```python
from build123d import *
from OCP.BRepFilletAPI import BRepFilletAPI_MakeChamfer

# Parameters (mm, degrees)
SKETCH2_W           = 152.4
SKETCH2_H           = 152.4
BOSS_EXTRUDE1_DEPTH = 25.4
BOSS_EXTRUDE2_DEPTH = 101.6
BOSS_EXTRUDE5_START = 50.8
BOSS_EXTRUDE5_DEPTH = 50.8
BOSS_EXTRUDE6_DEPTH = 25.4
SKETCH6_W           = 127
SKETCH6_H           = 98.02354915
CUT_EXTRUDE1_DEPTH  = 139.7
SKETCH7_R           = 8.255
CUT_EXTRUDE2_DEPTH  = 12.7
CHAMFER1_SIZE       = 7.62
CHAMFER1_SIZE2      = 2.773453185
FILLET1_R           = 12.7


with BuildPart() as part:
    # Sketch2 → Boss-Extrude1 (new body)
    with BuildSketch(Plane(origin=(0, 0, 0), x_dir=(1, 0, 0), z_dir=(0, 1, 0))):
        with BuildLine():
            Line((0, 76.2), (76.2, 76.2))
            Line((76.2, 76.2), (76.2, 123.42354915))
            ThreePointArc((76.2, 123.42354915), (44.823274072, 88.963087986), (0, 76.2))
        make_face()
        with BuildLine():
            Line((-76.2, 123.42354915), (-76.2, 76.2))
            Line((-76.2, 76.2), (0, 76.2))
            ThreePointArc((0, 76.2), (-44.823274072, 88.963087986), (-76.2, 123.42354915))
        make_face()
        Rectangle(SKETCH2_W, SKETCH2_H)
    extrude(amount=BOSS_EXTRUDE1_DEPTH)

    # Sketch3 → Boss-Extrude2 (add)
    with BuildSketch(Plane(origin=(0, 25.4, 0), x_dir=(1, 0, 0), z_dir=(0, 1, 0))):
        with BuildLine():
            ThreePointArc((76.2, 123.42354915), (0, 76.2), (-76.2, 123.42354915))
            Line((-76.2, 123.42354915), (-76.2, 98.02354915))
            ThreePointArc((-76.2, 98.02354915), (0, 60.787742764), (76.2, 98.02354915))
            Line((76.2, 98.02354915), (76.2, 123.42354915))
        make_face()
        with BuildLine():
            ThreePointArc((76.2, 78.97354915), (0, 46.95399651), (-76.2, 78.97354915))
            Line((-76.2, 78.97354915), (-76.2, -76.2))
            Line((-76.2, -76.2), (76.2, -76.2))
            Line((76.2, -76.2), (76.2, 78.97354915))
        make_face()
    extrude(amount=BOSS_EXTRUDE2_DEPTH)

    # Sketch5 → Boss-Extrude5 (add)
    with BuildSketch(Plane(origin=(0, 0, 0), x_dir=(1, 0, 0), z_dir=(0, 1, 0)).offset(BOSS_EXTRUDE5_START)):
        with BuildLine():
            Line((-76.2, 123.42354915), (-76.2, -76.2))
            Line((-76.2, -76.2), (76.2, -76.2))
            Line((76.2, -76.2), (76.2, 123.42354915))
            ThreePointArc((76.2, 123.42354915), (0, 76.2), (-76.2, 123.42354915))
        make_face()
    extrude(amount=BOSS_EXTRUDE5_DEPTH)

    # Sketch4 → Boss-Extrude6 (add)
    with BuildSketch(Plane(origin=(0, 127, 0), x_dir=(1, 0, 0), z_dir=(0, 1, 0))):
        with BuildLine():
            Line((-76.2, 123.42354915), (-76.2, -76.2))
            Line((-76.2, -76.2), (76.2, -76.2))
            Line((76.2, -76.2), (76.2, 123.42354915))
            ThreePointArc((76.2, 123.42354915), (0, 76.2), (-76.2, 123.42354915))
        make_face()
    extrude(amount=BOSS_EXTRUDE6_DEPTH)

    # Sketch6 → Cut-Extrude1 (cut)
    with BuildSketch(Plane(origin=(0, 152.4, 0), x_dir=(1, 0, 0), z_dir=(0, 1, 0))):
        with Locations((0, -14.488225425)):
            Rectangle(SKETCH6_W, SKETCH6_H)
    extrude(amount=-CUT_EXTRUDE1_DEPTH, mode=Mode.SUBTRACT)

    # Sketch7 → Cut-Extrude2 (cut)
    with BuildSketch(Plane(origin=(0, 12.7, 0), x_dir=(1, 0, 0), z_dir=(0, 1, 0))):
        with Locations(Location((-13.0048, -50.8, 0), (0, 0, 270))):
            Circle(SKETCH7_R)
        with Locations(Location((13.0048, -50.8, 0), (0, 0, 270))):
            Circle(SKETCH7_R)
    extrude(amount=-CUT_EXTRUDE2_DEPTH, mode=Mode.SUBTRACT)

    # Chamfer1: one chamfer whose edges measure the first distance from different faces: ONE call of the kernel's chamfer builder (chamfer() names one face for all edges)
    chamfer1_edges_1 = [part.edges().sort_by_distance(p)[0] for p in [
        (-13.0048, 0, 42.545),
    ]]
    chamfer1_side_1 = [part.faces().sort_by_distance(p)[0] for p in [
        (-13.0048, 6.35, 42.545),
    ]]
    chamfer1_edges_2 = [part.edges().sort_by_distance(p)[0] for p in [
        (13.0048, 0, 42.545),
    ]]
    chamfer1_side_2 = [part.faces().sort_by_distance(p)[0] for p in [
        (13.0048, 6.35, 42.545),
    ]]
    chamfer1 = BRepFilletAPI_MakeChamfer(part.part.solid().wrapped)
    for e in chamfer1_edges_1:
        chamfer1.Add(CHAMFER1_SIZE, CHAMFER1_SIZE2, e.wrapped, chamfer1_side_1[0].wrapped)  # the first distance lies on this face
    for e in chamfer1_edges_2:
        chamfer1.Add(CHAMFER1_SIZE, CHAMFER1_SIZE2, e.wrapped, chamfer1_side_2[0].wrapped)  # the first distance lies on this face
    add(Compound.cast(chamfer1.Shape()), mode=Mode.REPLACE)

    # Fillet1
    fillet1_edges = [part.edges().sort_by_distance(p)[0] for p in [
        (76.2, 76.2, 76.2),
        (-76.2, 76.2, 76.2),
        (76.2, 0, -23.611774575),
        (0, 0, 76.2),
        (-76.2, 0, -23.611774575),
    ]]
    fillet(fillet1_edges, radius=FILLET1_R)


solid = part.part
```
Verification items for the finished model (mm, model axes). A direction names the side the tool comes from. Give positions to 0.01 mm unless a question says otherwise; leave off trailing zeros. Order: outer loops, then holes, each group sorted by start corner. A loop starts at its lowest first (then second) coordinate and runs counter-clockwise, first axis right, second up. Notation, with made-up numbers: M 63.25,-10 L 76.25,-10 A22 ccw 76.25,1 Z; hole C 82.25,-29.5 d8. An arc over 180 degrees is marked long. Return JSON: item names as keys, results as strings. Group by question number.
1) Go/stop test with flat-tipped pins: pin 1 Ø12 at (x, z) = (34, 11) entering from +Y; pin 2 Ø1 at (x, y) = (20, 67.5) entering from -Z; pin 3 Ø10 at (x, z) = (-13, 50.8) entering from -Y. Record where each tip stops, or that it passes through.
2) Mould release check, pull along Y, two halves, no side actions. Record for faces 1 (the face through (-1, 152.4, -47)), 2 (the face through (-6, 101.6, -59)), 3 (the face through (72.38, 3.62, -31.27)): pulls with the +Y half, pulls with the -Y half, needs draft (parallel to the pull), parting line crosses it, or undercut.
3) Access from +Z, -Z, +X, -X, +Y, -Y to the whole of each face (thin tool, end or side, straight path). Record for faces 4 (the face through (-1, 84, -34.524)), 5 (the face through (-1.229, 37.922, -60.796)), 6 (the face through (1.32, 75.13, -76.21)).
4) Section check C-C on y = 61. Record the cut outline in (x, z).
5) Section check D-D on z = -10.5. Record the cut outline in (x, y).
6) Section check A-A on y = 44.5. Record the cut outline in (x, z).
7) Scan lines: line 1 (Z direction, x = 3, y = 96.5); line 2 (X direction, y = 129, z = 54); line 3 (Z direction, x = 30, y = 30). Record each from-to range of solid material in increasing order.
8) Section check B-B on z = 50.8. Record the cut outline in (x, y).
Answer block:
{
 "1": {"pin 1": "stops at y = 12.7", "pin 2": "stops at z = -78.71", "pin 3": "passes through"},
 "2": {"face 1": "pulls with the +Y half", "face 2": "undercut", "face 3": "pulls with the -Y half"},
 "3": {"face 4": "+Y", "face 5": "none", "face 6": "-Z, +Y, -Y"},
 "4": {"outline": "M -76.2,-123.42 A85.09 cw 76.2,-123.42 L 76.2,63.5 A12.7 ccw 63.5,76.2 L -63.5,76.2 A12.7 ccw -76.2,63.5 Z; hole M -63.5,-34.52 L 63.5,-34.52 L 63.5,63.5 L -63.5,63.5 Z"},
 "5": {"outline": "M -76.2,12.7 A12.7 ccw -63.5,0 L 63.5,0 A12.7 ccw 76.2,12.7 L 76.2,152.4 L 63.5,152.4 L 63.5,12.7 L -63.5,12.7 L -63.5,152.4 L -76.2,152.4 Z"},
 "6": {"outline": "M -76.2,-123.42 A85.09 cw 76.2,-123.42 L 76.2,-98.02 A96.59 ccw -76.2,-98.02 Z; M -76.2,-78.97 A106.68 cw 76.2,-78.97 L 76.2,63.5 A12.7 ccw 63.5,76.2 L -63.5,76.2 A12.7 ccw -76.2,63.5 Z; hole M -63.5,-34.52 L 63.5,-34.52 L 63.5,63.5 L -63.5,63.5 Z"},
 "7": {"line 1": "z = -76.25 to -34.52, 63.5 to 76.2", "line 2": "x = -76.2 to -63.5, 63.5 to 76.2", "line 3": "z = -81.66 to -65.56, -51.26 to -34.52, 63.5 to 76.2"},
 "8": {"outline": "M -76.2,12.7 A12.7 ccw -63.5,0 L -24.03,0 L -21.26,7.62 L -21.26,12.7 L -63.5,12.7 L -63.5,152.4 L -76.2,152.4 Z; M -4.75,7.62 L -1.98,0 L 1.98,0 L 4.75,7.62 L 4.75,12.7 L -4.75,12.7 Z; M 21.26,7.62 L 24.03,0 L 63.5,0 A12.7 ccw 76.2,12.7 L 76.2,152.4 L 63.5,152.4 L 63.5,12.7 L 21.26,12.7 Z"}
}
